Autodesk Inventor part; units mm, degrees
ref_plane "YZ Plane" through (0, 0, 0) normal (1, 0, 0) x (0, 1, 0)
ref_plane "XZ Plane" through (0, 0, 0) normal (0, 1, 0) x (-1, 0, 0)
ref_plane "XY Plane" through (0, 0, 0) normal (0, 0, 1) x (1, 0, 0)
sketch "Sketch1" plane through (0, 0, 0) normal (1, 0, 0) x (0, 1, 0)
  line L0 (-4.5658, 12.6718) -> (-17.2658, 12.6718)
  line L1 (-23.6158, 6.3218) -> (-23.6158, -82.5782)
  line L2 (-17.2658, -88.9282) -> (-4.5658, -88.9282)
  line L3 (1.7842, -82.5782) -> (1.7842, 6.3218)
  arc A0 (1.7842, 6.3218) -> (-4.5658, 12.6718) centre (-4.5658, 6.3218) ccw
  arc A1 (-17.2658, 12.6718) -> (-23.6158, 6.3218) centre (-17.2658, 6.3218) ccw
  arc A2 (-23.6158, -82.5782) -> (-17.2658, -88.9282) centre (-17.2658, -82.5782) ccw
  arc A3 (-4.5658, -88.9282) -> (1.7842, -82.5782) centre (-4.5658, -82.5782) ccw
  point P0 (0, 0)
  point P1 (1.7842, 12.6718)
  point P2 (-23.6158, -88.9282)
  point P3 (-23.6158, 12.6718)
  point P4 (1.7842, -88.9282)
  dimension "d0" = 25.4
  dimension "d1" = 101.6
  dimension "d4" = 6.35
extrude "Extrusion1" add sketch "Sketch1" along normal blind 4.064
sketch "Sketch2" plane through (4.064, 0, 0) normal (1, 0, 0) x (0, 0, -1)
  arc A0 (82.5782, -23.6158) -> (88.9282, -17.2658) centre (82.5782, -17.2658) ccw
  line L0 (-12.6718, -4.5658) -> (-12.6718, -17.2658)
  line L1 (82.5782, 1.7842) -> (-6.3218, 1.7842)
  line L2 (82.5782, -1.213) -> (-6.3218, -1.213)
  line L3 (-6.3218, -20.6186) -> (82.5782, -20.6186)
  line L4 (-6.3218, -20.6186) -> (82.5782, -20.6186)
  line L5 (82.5782, -20.6186) -> (82.5782, -23.6158)
  line L6 (82.5782, -23.6158) -> (-6.3218, -23.6158)
  line L7 (-6.3218, -23.6158) -> (-6.3218, -20.6186)
  line L8 (-6.3218, -1.213) -> (82.5782, -1.213)
  line L9 (82.5782, -1.213) -> (82.5782, 1.7842)
  line L10 (82.5782, 1.7842) -> (-6.3218, 1.7842)
  line L11 (-6.3218, 1.7842) -> (-6.3218, -1.213)
  point P0 (0, 0)
  dimension "d6" = 19.4056
extrude "Extrusion2" add sketch "Sketch2" along normal blind 25.4
sketch "Sketch3" plane through (4.064, -1.213, 6.3218) normal (0, 0, 1) x (1, 0, 0)
  line L0 (25.4, 2.9972) -> (25.4, 0)
  line L1 (25.4, 2.9972) -> (25.4, 0)
  line L2 (25.4, -19.4056) -> (25.4, -22.4028)
  line L3 (25.4, -22.4028) -> (29.8318, -19.2996)
  line L4 (25.4, -19.4056) -> (25.4, -22.4028)
  line L5 (0, 2.9972) -> (25.4, 2.9972)
  line L6 (25.4, 2.9972) -> (25.4, 0)
  line L7 (25.4, 2.9972) -> (29.8318, -0.106)
  line L8 (29.7989, -0.0829) -> (25.4, 0)
  line L9 (29.8318, -19.2996) -> (25.4, -19.4056)
  point P0 (-4.064, 1.213)
  dimension "d35" = 5.4102
  dimension "d36" = 55
  dimension "d37" = 5.4102
  dimension "d38" = 55
sketch "Sketch4" plane through (0, 0, 0) normal (-1, 0, 0) x (0, 0, 1)
  arc A0 (12.6718, -4.5658) -> (6.3218, 1.7842) centre (6.3218, -4.5658) ccw
  line L0 (-5.4816, 0) -> (-17.3349, 0)
  line L1 (-17.3349, 0) -> (-17.3349, -4.7413)
  line L2 (-17.3349, -4.7413) -> (-5.4816, -4.7413)
  line L3 (-5.4816, -4.7413) -> (-5.4816, 0)
  line L4 (-30.9663, 0) -> (-19.1129, 0)
  line L5 (-19.1129, 0) -> (-19.1129, -4.7413)
  line L6 (-19.1129, -4.7413) -> (-30.9663, -4.7413)
  line L7 (-30.9663, -4.7413) -> (-30.9663, 0)
  line L8 (-32.7443, 0) -> (-44.5976, 0)
  line L9 (-44.5976, -4.7413) -> (-32.7443, -4.7413)
  line L10 (-32.7443, -4.7413) -> (-32.7443, 0)
  line L11 (-44.5976, 0) -> (-44.5976, -4.7413)
  arc A1 (-82.5782, 1.7842) -> (-88.9282, -4.5658) centre (-82.5782, -4.5658) ccw
  line L12 (-58.2289, -4.7413) -> (-58.2289, 0)
  line L13 (-58.2289, 0) -> (-46.3756, 0)
  line L14 (-46.3756, -4.7413) -> (-58.2289, -4.7413)
  line L15 (-46.3756, 0) -> (-46.3756, -4.7413)
  line L16 (-60.0069, 0) -> (-71.8603, 0)
  line L17 (-71.8603, 0) -> (-71.8603, -4.7413)
  line L18 (-71.8603, -4.7413) -> (-60.0069, -4.7413)
  line L19 (-60.0069, -4.7413) -> (-60.0069, 0)
  line L20 (-85.4916, 0) -> (-73.6383, 0)
  line L21 (-73.6383, 0) -> (-73.6383, -4.7413)
  line L22 (-85.4916, -4.7413) -> (-85.4916, 0)
  line L23 (-73.6383, -4.7413) -> (-85.4916, -4.7413)
  line L24 (-3.7036, 0) -> (8.1497, 0)
  line L25 (8.1497, 0) -> (8.1497, -4.7413)
  line L26 (8.1497, -4.7413) -> (-3.7036, -4.7413)
  line L27 (-3.7036, -4.7413) -> (-3.7036, 0)
  point P0 (0, 0)
  dimension "d47" = 1.778
extrude "Extrusion4" add sketch "Sketch4" along normal blind 50.8
extrude "Extrusion6" add sketch "Sketch3" against normal up to surface (88.9 mm away)
sketch "Sketch8" plane through (0, -23.6158, -82.5782) normal (0, -1, 0) x (1, 0, 0)
  point P0 (0, 82.5782)
sketch "Sketch9" plane through (0, -23.6158, -82.5782) normal (0, -1, 0) x (1, 0, 0)
  line L0 (29.0881, 73.7677) -> (29.0881, 12.702) construction
  line L1 (29.0881, 12.702) -> (2.3767, 12.702) construction
  line L2 (2.3767, 12.702) -> (2.3767, 73.7677) construction
  line L3 (2.3767, 73.7677) -> (29.0881, 73.7677) construction
  point P0 (0, 82.5782)
emboss "Emboss2" [suppressed]
sketch "Sketch10" plane through (4.064, 0, 0) normal (1, 0, 0) x (0, 0, -1)
  line L0 (-6.3218, -20.6186) -> (82.5782, -20.6186)
  line L1 (82.5782, 1.7842) -> (82.5782, -1.213)
  line L2 (-6.3218, -1.213) -> (-6.3218, 1.7842)
  line L3 (82.5782, -1.213) -> (-6.3218, -1.213)
  line L4 (-6.3218, -20.6186) -> (82.5782, -20.6186)
  line L5 (82.5782, -20.6186) -> (87.9709, -20.6186)
  arc A0 (82.5782, -23.6158) -> (88.9282, -17.2658) centre (82.5782, -17.2658) ccw
  line L6 (82.5782, -1.213) -> (87.9709, -1.213)
  arc A1 (88.9282, -4.5658) -> (82.5782, 1.7842) centre (82.5782, -4.5658) ccw
  line L7 (-6.3218, -20.6186) -> (82.5782, -20.6186)
  line L8 (-6.3218, -20.6186) -> (-11.7145, -20.6186)
  arc A2 (-12.6718, -17.2658) -> (-6.3218, -23.6158) centre (-6.3218, -17.2658) ccw
  line L9 (-6.3218, -1.213) -> (-11.7145, -1.213)
  line L10 (87.9709, -1.213) -> (88.9282, -1.213)
  line L11 (88.9282, -1.213) -> (88.9282, -20.6186)
  line L12 (88.9282, -20.6186) -> (87.9709, -20.6186)
  line L13 (-11.7145, -20.6186) -> (-12.6718, -20.6186)
  line L14 (-12.6718, -20.6186) -> (-12.6718, -1.213)
  line L15 (-12.6718, -1.213) -> (-11.7145, -1.213)
  arc A3 (-6.3218, 1.7842) -> (-12.6718, -4.5658) centre (-6.3218, -4.5658) ccw
  point P0 (0, 0)
  point P1 (42.8061, -20.6186)
  point P2 (29.4692, -20.6186)
  point P3 (42.8061, -20.6186)
extrude "Extrusion7" cut sketch "Sketch10" against normal blind 2.032 contours L8 A2 L14 A3 L9 L3 L6 A1 L11 A0 L5 L0 | L13 L14 A2 | A0 L11 L12 | L14 L15 A3 | A1 L10 L11
properties part number "the whole thing"
Could you check a few things on this model? Use its own coordinates, in mm. A direction names the side the tool comes from. Round coordinates to 2 decimals unless told otherwise and drop trailing zeros. Write each loop counter-clockwise with the first axis right and the second up, starting at its lowest first coordinate (ties: lowest second). Pieces come first, ordered by that corner, then holes. Notation, with made-up numbers: M 57.5,24.25 L 107.5,24.25 A36 cw 107.5,58.25 Z; hole C 11,24 d2. An arc over 180 degrees is marked long. Answer in a Markdown table with one row per item. Add a question column.
Q1. If we mould it in two halves opening along Y, with no side actions, what happens to faces 4 (the flat face through (16, -20.619, -39)), 5 (the flat face through (-25, -2, -17.335)), 6 (the flat face through (-25, -4.741, 2))? For each: +Y half, -Y half, draft (parallel to the pull), parting line (faces both ways), or undercut.
Q2. Imagine slicing it at A-A (x = 16). Please give me the cut outline in (y, z).
Q3. If I drill on line 1 (Y direction, x = 15, z = -18.5); line 2 (X direction, y = -2.75, z = -2); line 3 (X direction, y = -15.75, z = -45.5), over which ranges is the centre line in solid material (lowest first)? Write a range as from..to.
Q4. Will these pins go through, and if not, where does the flat tip stop? pin 1 Ø5 at (x, y) = (-37.5, -1.5) entering from +Z; pin 2 Ø13 at (x, z) = (-26, 1.5) entering from -Y; pin 3 Ø1.5 at (y, z) = (1, -85.5) entering from +X.
Q5. On a 3-axis mill with a long thin cutter (end or side, diameter ignored), from which of +Z, -Z, +X, -X, +Y, -Y can I reach the whole of each face in a straight line? I mean faces 1 (the flat face through (4.064, -22, -85)), 2 (the flat face through (-25, -4.741, -52)), 3 (the flat face through (-25, -2, -5.482)). Say none if no direction works.
Q6. Imagine slicing it at B-B (x = -12). Please give me the cut outline in (y, z), then the cut area to 3 significant figures.
Q7. Imagine slicing it at D-D (y = -6.25). Please give me the cut outline in (x, z), then the cut area to 3 significant figures.
Q8. Imagine slicing it at C-C (z = -8). Please give me the cut outline in (x, y).
Values:
| question | item | result |
|---|---|---|
| 1 | face 4 | undercut |
| 1 | face 5 | draft |
| 1 | face 6 | -Y half |
| 2 | outline | M -23.62,-82.58 L -20.62,-82.58 L -20.62,6.32 L -23.62,6.32 Z; M -1.21,-82.58 L 1.78,-82.58 L 1.78,6.32 L -1.21,6.32 Z |
| 3 | line 1 | -23.62..-20.62, -1.21..1.78 |
| 3 | line 2 | -50.8..2.03 |
| 3 | line 3 | 0..2.03 |
| 4 | pin 1 | z = 8.15 |
| 4 | pin 2 | y = -4.74 |
| 4 | pin 3 | x = 4.06 |
| 5 | face 1 | -Z, +X, +Y, -Y |
| 5 | face 2 | +Z, -Z, -X, -Y |
| 5 | face 3 | -X, +Y, -Y |
| 6 | outline | M -4.74,-85.49 L 0,-85.49 L 0,-73.64 L -4.74,-73.64 Z; M -4.74,-71.86 L 0,-71.86 L 0,-60.01 L -4.74,-60.01 Z; M -4.74,-58.23 L 0,-58.23 L 0,-46.38 L -4.74,-46.38 Z; M -4.74,-44.6 L 0,-44.6 L 0,-32.74 L -4.74,-32.74 Z; M -4.74,-30.97 L 0,-30.97 L 0,-19.11 L -4.74,-19.11 Z; M -4.74,-17.33 L 0,-17.33 L 0,-5.48 L -4.74,-5.48 Z; M -4.74,-3.7 L 0,-3.7 L 0,8.15 L -4.74,8.15 Z |
| 6 | area | 393 mm^2 |
| 7 | outline | M 0,-88.93 L 2.03,-88.93 L 2.03,12.67 L 0,12.67 Z |
| 7 | area | 206 mm^2 |
| 8 | outline | M -50.8,-4.74 L 0,-4.74 L 0,-23.62 L 29.46,-23.62 L 33.9,-20.51 L 29.46,-20.62 L 2.03,-20.62 L 2.03,-1.21 L 29.46,-1.21 L 33.86,-1.3 L 29.46,1.78 L 0,1.78 L 0,0 L -50.8,0 Z |
